from build123d import *

# Parameters (mm, degrees)
SKETCH1_W           = 40
SKETCH1_H           = 20
BOSS_EXTRUDE1_DEPTH = 3.3
BOSS_EXTRUDE2_DEPTH = 1.5
SKETCH3_R           = 2.45
CUT_EXTRUDE1_DEPTH  = 2
BOSS_EXTRUDE3_DEPTH = 5.05
SKETCH5_R           = 0.9
CUT_EXTRUDE2_DEPTH  = 4


with BuildPart() as part:
    # Sketch1 → Boss-Extrude1 (new body)
    with BuildSketch(Plane(origin=(0, 0, 0), x_dir=(1, 0, 0), z_dir=(0, 1, 0))):
        Rectangle(SKETCH1_W, SKETCH1_H)
    extrude(amount=BOSS_EXTRUDE1_DEPTH)

    # Sketch2 → Boss-Extrude2 (add)
    with BuildSketch(Plane(origin=(0, 3.3, 0), x_dir=(1, 0, 0), z_dir=(0, 1, 0))):
        with BuildLine():
            Line((-19, 7.5), (-19, -7.5))
            ThreePointArc((-19, -7.5), (-18.560660172, -8.560660172), (-17.5, -9))
            Line((-17.5, -9), (17.5, -9))
            ThreePointArc((17.5, -9), (18.560660172, -8.560660172), (19, -7.5))
            Line((19, -7.5), (19, 7.5))
            ThreePointArc((19, 7.5), (18.560660172, 8.560660172), (17.5, 9))
            Line((17.5, 9), (-17.5, 9))
            ThreePointArc((-17.5, 9), (-18.560660172, 8.560660172), (-19, 7.5))
        make_face()
        with BuildLine():
            Line((-18.4, 6.3), (-18.4, -6.3))
            ThreePointArc((-18.4, -6.3), (-16.439339828, -6.439339828), (-16.3, -8.4))
            Line((-16.3, -8.4), (16.3, -8.4))
            ThreePointArc((16.3, -8.4), (16.439339828, -6.439339828), (18.4, -6.3))
            Line((18.4, -6.3), (18.4, 6.3))
            ThreePointArc((18.4, 6.3), (16.439339828, 6.439339828), (16.3, 8.4))
            Line((16.3, 8.4), (-16.3, 8.4))
            ThreePointArc((-16.3, 8.4), (-16.439339828, 6.439339828), (-18.4, 6.3))
        make_face(mode=Mode.SUBTRACT)
    extrude(amount=BOSS_EXTRUDE2_DEPTH)

    # Sketch3 → Cut-Extrude1 (cut)
    with BuildSketch(Plane(origin=(0, 3.3, 0), x_dir=(-1, 0, 0), z_dir=(0, 1, 0))):
        with Locations((10.52883238, 0)):
            Circle(SKETCH3_R)
    extrude(amount=-CUT_EXTRUDE1_DEPTH, mode=Mode.SUBTRACT)

    # Sketch4 → Boss-Extrude3 (add)
    with BuildSketch(Plane(origin=(0, 3.3, 0), x_dir=(1, 0, 0), z_dir=(0, 1, 0))):
        with BuildLine():
            Line((-15.52883238, -5), (-7.02883238, -5))
            Line((-7.02883238, -5), (-7.02883238, -6.3))
            Line((-7.02883238, -6.3), (-8.729526959, -6.3))
            ThreePointArc((-8.729526959, -6.3), (-10.52883238, -8.15), (-12.328137802, -6.3))
            Line((-12.328137802, -6.3), (-15.82883238, -6.3))
            ThreePointArc((-15.82883238, -6.3), (-16.535939162, -6.007106781), (-16.82883238, -5.3))
            Line((-16.82883238, -5.3), (-16.82883238, -1.25))
            ThreePointArc((-16.82883238, -1.25), (-18.07883238, 0), (-16.82883238, 1.25))
            Line((-16.82883238, 1.25), (-16.82883238, 5.3))
            ThreePointArc((-16.82883238, 5.3), (-16.535939162, 6.007106781), (-15.82883238, 6.3))
            Line((-15.82883238, 6.3), (-12.328137802, 6.3))
            ThreePointArc((-12.328137802, 6.3), (-10.52883238, 8.15), (-8.729526959, 6.3))
            Line((-8.729526959, 6.3), (-7.02883238, 6.3))
            Line((-7.02883238, 6.3), (-7.02883238, 5))
            Line((-7.02883238, 5), (-15.52883238, 5))
            Line((-15.52883238, 5), (-15.52883238, -5))
        make_face()
    extrude(amount=BOSS_EXTRUDE3_DEPTH)

    # Sketch5 → Cut-Extrude2 (cut)
    with BuildSketch(Plane(origin=(0, 8.35, 0), x_dir=(-1, 0, 0), z_dir=(0, 1, 0))):
        with Locations((10.52883238, 6.35)):
            Circle(SKETCH5_R)
        with Locations((10.52883238, -6.35)):
            Circle(SKETCH5_R)
    extrude(amount=-CUT_EXTRUDE2_DEPTH, mode=Mode.SUBTRACT)


solid = part.part
CAD build for the part. Positions are in the model's coordinates, mm. A direction names the side the tool comes from. Give positions to 0.01 mm unless a question says otherwise; leave off trailing zeros. Order: outer loops, then holes, each group sorted by start corner. A loop starts at its lowest first (then second) coordinate and runs counter-clockwise, first axis right, second up. Notation, with made-up numbers: (8, -35.75) -> (52, -35.75) arc R3 ccw to (52, -30.75) -> close; hole circle Ø8 at (-37, 26). An arc over 180 degrees is marked (long way). Return JSON: item names as keys, results as strings.
Q1. Drill centre lines: line 1 (X direction, y = 4.25, z = 3.25); line 2 (Z direction, x = -13.5, y = 6); line 3 (X direction, y = 5.5, z = -1.5). Where is each one in solid material? Low to high.
Working result:
{"line 1": "-19 to -18.4, -16.83 to -15.53, 18.4 to 19", "line 2": "-6.3 to -5, 5 to 6.3", "line 3": "-16.83 to -15.53"}
Q2. Which spindle directions (+Z, -Z, +X, -X, +Y, -Y) get a long thin tool onto all of the face, cutting with end or side? Do faces 4 (the face through (0, 2, -10)), 5 (the face through (-7.029, 6, 6)). Say none if no direction does.
Working result:
{"face 4": "-Z, +X, -X, +Y, -Y", "face 5": "+Y"}
Q3. Mould opens along X. For faces 1 (the face through (0, 4, -9)), 2 (the face through (-16.544, 5.79, -5.999)), 3 (the face through (20, 2, 0)) say: pulls with the +X half, pulls with the -X half, needs draft (parallel to the pull), parting line crosses it, or undercut.
Working result:
{"face 1": "needs draft", "face 2": "undercut", "face 3": "pulls with the +X half"}
Q4. Saw through at C-C (z = 4.5). Write the cut outline in (x, y).
Working result:
{"outline": "(-20, 0) -> (20, 0) -> (20, 3.3) -> (19, 3.3) -> (19, 4.8) -> (18.4, 4.8) -> (18.4, 3.3) -> (-15.53, 3.3) -> (-15.53, 8.35) -> (-16.83, 8.35) -> (-16.83, 3.3) -> (-18.4, 3.3) -> (-18.4, 4.8) -> (-19, 4.8) -> (-19, 3.3) -> (-20, 3.3) -> close"}
Q5. Saw through at A-A (x = -0.5). Write the cut outline in (y, z), then the cut area to 3 significant figures.
Working result:
{"outline": "(0, -10) -> (3.3, -10) -> (3.3, -9) -> (4.8, -9) -> (4.8, -8.4) -> (3.3, -8.4) -> (3.3, 8.4) -> (4.8, 8.4) -> (4.8, 9) -> (3.3, 9) -> (3.3, 10) -> (0, 10) -> close", "area": "67.8 mm²"}
Q6. Saw through at D-D (z = 0). Write the cut outline in (x, y).
Working result:
{"outline": "(-20, 0) -> (20, 0) -> (20, 3.3) -> (19, 3.3) -> (19, 4.8) -> (18.4, 4.8) -> (18.4, 3.3) -> (-8.08, 3.3) -> (-8.08, 1.3) -> (-12.98, 1.3) -> (-12.98, 3.3) -> (-15.53, 3.3) -> (-15.53, 8.35) -> (-18.08, 8.35) -> (-18.08, 3.3) -> (-18.4, 3.3) -> (-18.4, 4.8) -> (-19, 4.8) -> (-19, 3.3) -> (-20, 3.3) -> close"}
Q7. Flat gauge pins, fed straight in: pin 1 (1.2 mm diameter, centred on y = 6.5, z = -3, fed in from -X); pin 2 (6 mm diameter, centred on x = 1.5, z = -4, fed in from +Y); pin 3 (0.8 mm diameter, centred on y = 4.5, z = -3.5, fed in from -X). Where does each tip first touch, or does it go through?
Working result:
{"pin 1": "x = -16.83", "pin 2": "y = 3.3", "pin 3": "x = -19"}
Q8. Saw through at B-B (y = 7). Write the cut outline in (x, z).
Working result:
{"outline": "(-16.83, -5.3) arc R1 ccw to (-15.83, -6.3) -> (-12.33, -6.3) arc R1.8 ccw (long way) to (-8.73, -6.3) -> (-7.03, -6.3) -> (-7.03, -5) -> (-15.53, -5) -> (-15.53, 5) -> (-7.03, 5) -> (-7.03, 6.3) -> (-8.73, 6.3) arc R1.8 ccw (long way) to (-12.33, 6.3) -> (-15.83, 6.3) arc R1 ccw to (-16.83, 5.3) -> (-16.83, 1.25) arc R1.25 ccw to (-16.83, -1.25) -> close; hole circle Ø1.8 at (-10.53, -6.35); hole circle Ø1.8 at (-10.53, 6.35)"}
